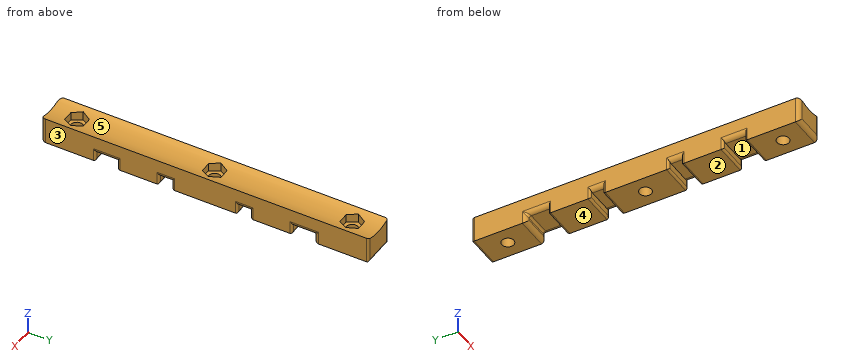
```python
from build123d import *

# Parameters (mm, degrees)
SKETCH_W        = 15
SKETCH_H        = 150
SKETCH_R        = 2.75
PAD_DEPTH       = 12
SKETCH003_W     = 10
SKETCH003_H     = 4
SKETCH003_W_2   = 6
POCKET002_DEPTH = 15.001
SKETCH004_R     = 20
POCKET003_DEPTH = 150.001
POCKET_DEPTH    = 5
FILLET_R        = 2
FILLET001_R     = 2
FILLET002_R     = 1
FILLET003_R     = 1
FILLET004_R     = 1
FILLET005_R     = 1
FILLET006_R     = 1
FILLET007_R     = 2


with BuildPart() as part:
    # Sketch → Pad (new body)
    with BuildSketch(Plane.XY):
        with Locations((7.5, 75)):
            Rectangle(SKETCH_W, SKETCH_H)
        with Locations((7.5, 138)):
            Circle(SKETCH_R, mode=Mode.SUBTRACT)
        with Locations((7.5, 75)):
            Circle(SKETCH_R, mode=Mode.SUBTRACT)
        with Locations((7.5, 12)):
            Circle(SKETCH_R, mode=Mode.SUBTRACT)
    extrude(amount=PAD_DEPTH)

    # Sketch003 → Pocket002 (cut, through all)
    with BuildSketch(Plane.YZ):
        with Locations((30, 2)):
            Rectangle(SKETCH003_W, SKETCH003_H)
        with Locations((57, 2)):
            Rectangle(SKETCH003_W_2, SKETCH003_H)
        with Locations((120, 2)):
            Rectangle(SKETCH003_W, SKETCH003_H)
        with Locations((93, 2)):
            Rectangle(SKETCH003_W_2, SKETCH003_H)
    extrude(amount=POCKET002_DEPTH, mode=Mode.SUBTRACT)

    # Sketch004 → Pocket003 (cut, through all)
    with BuildSketch(Plane.XZ):
        with Locations((7.5, 30.540496)):
            Circle(SKETCH004_R)
    extrude(amount=-POCKET003_DEPTH, mode=Mode.SUBTRACT)

    # Sketch005 → Pocket (cut)
    with BuildSketch(Plane.XY.offset(12)):
        Polygon((9.953739, 133.75), (12.407477, 138), (9.953739, 142.25), (5.046261, 142.25), (2.592523, 138), (5.046261, 133.75), align=None)
        Polygon((9.953739, 70.75), (12.407477, 75), (9.953739, 79.25), (5.046261, 79.25), (2.592523, 75), (5.046261, 70.75), align=None)
        Polygon((9.953739, 16.25), (5.046261, 16.25), (2.592523, 12), (5.046261, 7.75), (9.953739, 7.75), (12.407477, 12), align=None)
    extrude(amount=-POCKET_DEPTH, mode=Mode.SUBTRACT)

    # Fillet
    fillet_edges = [part.edges().sort_by_distance(p)[0] for p in [
        (15, 120, 4),
        (0, 120, 4),
        (15, 93, 4),
        (0, 93, 4),
        (15, 57, 4),
        (0, 57, 4),
        (15, 30, 4),
        (0, 30, 4),
    ]]
    fillet(fillet_edges, radius=FILLET_R)

    # Fillet001
    fillet001_edges = [part.edges().sort_by_distance(p)[0] for p in [
        (15, 125, 2),
        (7.5, 125, 0),
        (0, 125, 2),
    ]]
    fillet(fillet001_edges, radius=FILLET001_R)

    # Fillet002
    fillet002_edges = [part.edges().sort_by_distance(p)[0] for p in [
        (7.5, 125, 4),
    ]]
    fillet(fillet002_edges, radius=FILLET002_R)

    # Fillet003
    fillet003_edges = [part.edges().sort_by_distance(p)[0] for p in [
        (0, 25, 2),
        (7.5, 25, 0),
        (15, 25, 2),
    ]]
    fillet(fillet003_edges, radius=FILLET003_R)

    # Fillet004
    fillet004_edges = [part.edges().sort_by_distance(p)[0] for p in [
        (0, 54, 2),
        (7.5, 54, 0),
        (15, 54, 2),
        (0, 90, 2),
        (7.5, 90, 0),
        (15, 90, 2),
        (0, 115, 2),
        (7.5, 115, 0),
        (15, 115, 2),
    ]]
    fillet(fillet004_edges, radius=FILLET004_R)

    # Fillet005
    fillet005_edges = [part.edges().sort_by_distance(p)[0] for p in [
        (15, 96, 2),
        (7.5, 96, 0),
        (0, 96, 2),
        (15, 60, 2),
        (7.5, 60, 0),
        (0, 60, 2),
        (15, 35, 2),
        (7.5, 35, 0),
        (0, 35, 2),
    ]]
    fillet(fillet005_edges, radius=FILLET005_R)

    # Fillet006
    fillet006_edges = [part.edges().sort_by_distance(p)[0] for p in [
        (15, 150, 6),
        (7.5, 150, 0),
        (0, 150, 6),
    ]]
    fillet(fillet006_edges, radius=FILLET006_R)

    # Fillet007
    fillet007_edges = [part.edges().sort_by_distance(p)[0] for p in [
        (0, 0, 6),
        (7.5, 0, 0),
        (15, 0, 6),
    ]]
    fillet(fillet007_edges, radius=FILLET007_R)


solid = part.part
```
Verification items for the finished model (mm, model axes). Face numbers are marked on the shaded views. A direction names the side the tool comes from. Give positions to 0.01 mm unless a question says otherwise; leave off trailing zeros. Order: outer loops, then holes, each group sorted by start corner. A loop starts at its lowest first (then second) coordinate and runs counter-clockwise, first axis right, second up. Notation, with made-up numbers: M 68.5,-21.5 L 117.5,-21.5 A6 ccw 117.5,-16.5 Z; hole C 19.5,66.25 d7. An arc over 180 degrees is marked long. Return JSON: item names as keys, results as strings. Group by question number.
1) Section check C-C on y = 57. Record the cut outline in (x, z).
2) Scan lines: line 1 (Y direction, x = 9.5, z = 10.25); line 2 (X direction, y = 12, z = 5.75); line 3 (Z direction, x = 4.75, y = 72.5). Record each from-to range of solid material in increasing order.
3) Section check B-B on x = 7.5. Give the number of separate pieces and of enclosed holes in the cut face, and give its area (3 significant figures).
4) Access from +Z, -Z, +X, -X, +Y, -Y to the whole of each face (thin tool, end or side, straight path). Record for the marked faces 1 and 2.
5) Section check A-A on y = 10.5. Record the cut outline in (x, z), and give its area (3 significant figures).
6) Mould release check, pull along X, two halves, no side actions. Record for the marked faces 3, 4 and 5: pulls with the +X half, pulls with the -X half, needs draft (parallel to the pull), parting line crosses it, or undercut.
7) Go/stop test with flat-tipped pins: pin 1 Ø8 at (x, y) = (6, 29.5) entering from -Z; pin 2 Ø7 at (x, y) = (7, 73.5) entering from +Z; pin 3 Ø9 at (x, y) = (7.5, 12) entering from +Z. Record where each tip stops, or that it passes through.
Answer block:
{
 "1": {"outline": "M 0,6 A2 ccw 2,4 L 13,4 A2 ccw 15,6 L 15,12 A20 cw 0,12 Z"},
 "2": {"line 1": "y = 0 to 7.75, 16.25 to 70.75, 79.25 to 133.75, 142.25 to 150", "line 2": "x = 0 to 4.75, 10.25 to 15", "line 3": "z = 0 to 7"},
 "3": {"separate pieces": "4", "enclosed holes": "0", "area": "1,240 mm^2"},
 "4": {"face 1": "-Z, +X, -X", "face 2": "-Z, +X, -X, +Y, -Y"},
 "5": {"outline": "M 0,0 L 5.2,0 L 5.2,7 L 3.46,7 L 3.46,10.95 A20 cw 0,12 Z; M 9.8,0 L 15,0 L 15,12 A20 cw 11.54,10.95 L 11.54,7 L 9.8,7 Z", "area": "103 mm^2"},
 "6": {"face 3": "pulls with the +X half", "face 4": "needs draft", "face 5": "undercut"},
 "7": {"pin 1": "stops at z = 4", "pin 2": "stops at z = 10.94", "pin 3": "stops at z = 11.04"}
}
